Build history of the part. All positions in model axes, mm. Round coordinates to 2 decimals unless told otherwise and drop trailing zeros. Write each loop counter-clockwise with the first axis right and the second up, starting at its lowest first coordinate (ties: lowest second). Pieces come first, ordered by that corner, then holes. Notation, with made-up numbers: (-21.75, -9) -> (20.25, -9) arc R24 ccw to (20.25, 11) -> close; hole circle Ø11 at (67.5, -34.5). An arc over 180 degrees is marked (long way). One line per question, with ' | ' between items.
from build123d import *

# Parameters (mm, degrees)
SKETCH2_R           = 2.4892
SKETCH2_R_2         = 2.489199995
SKETCH2_R_3         = 2.489199998
BOSS_EXTRUDE1_DEPTH = 2.286
FILLET6_R           = 12.7
FILLET7_R           = 15.24


with BuildPart() as part:
    # Sketch2 → Boss-Extrude1 (new body)
    with BuildSketch(Plane.XY):
        Polygon((33.430156219, 560.153270419), (33.430156219, 610.953270419), (-17.369843781, 610.953270419), (-70.882869838, 630.430419049), (-92.601148921, 570.759937623), (-96.944804753, 558.825841343), (-49.208419617, 541.451218062), (-17.464279743, 534.753270419), (33.335720257, 534.753270419), (33.335720257, 547.453270419), align=None)
        with Locations((-4.764279743, 566.503270419)):
            Circle(SKETCH2_R, mode=Mode.SUBTRACT)
        with Locations((-4.764279743, 579.203270419)):
            Circle(SKETCH2_R, mode=Mode.SUBTRACT)
        with Locations((7.935720257, 566.503270419)):
            Circle(SKETCH2_R, mode=Mode.SUBTRACT)
        with Locations((20.635720257, 566.503270419)):
            Circle(SKETCH2_R, mode=Mode.SUBTRACT)
        with Locations((7.935720257, 579.203270419)):
            Circle(SKETCH2_R, mode=Mode.SUBTRACT)
        with Locations((20.635720257, 579.203270419)):
            Circle(SKETCH2_R, mode=Mode.SUBTRACT)
        with Locations((-4.764279743, 591.903270419)):
            Circle(SKETCH2_R, mode=Mode.SUBTRACT)
        with Locations((-4.764279743, 604.603270419)):
            Circle(SKETCH2_R, mode=Mode.SUBTRACT)
        with Locations((7.935720257, 591.903270419)):
            Circle(SKETCH2_R, mode=Mode.SUBTRACT)
        with Locations((20.635720257, 591.903270419)):
            Circle(SKETCH2_R, mode=Mode.SUBTRACT)
        with Locations((7.935720257, 604.603270419)):
            Circle(SKETCH2_R, mode=Mode.SUBTRACT)
        with Locations((20.635720257, 604.603270419)):
            Circle(SKETCH2_R, mode=Mode.SUBTRACT)
        with Locations((20.635720257, 553.803270419)):
            Circle(SKETCH2_R, mode=Mode.SUBTRACT)
        with Locations((-4.764279743, 553.803270419)):
            Circle(SKETCH2_R, mode=Mode.SUBTRACT)
        with Locations((7.935720257, 553.803270419)):
            Circle(SKETCH2_R, mode=Mode.SUBTRACT)
        with Locations((20.635720257, 541.103270419)):
            Circle(SKETCH2_R, mode=Mode.SUBTRACT)
        with Locations((7.935720257, 541.103270419)):
            Circle(SKETCH2_R, mode=Mode.SUBTRACT)
        with Locations((-4.764279743, 541.103270419)):
            Circle(SKETCH2_R, mode=Mode.SUBTRACT)
        with Locations((-37.25240889, 611.432403444)):
            Circle(SKETCH2_R, mode=Mode.SUBTRACT)
        with Locations((-50.283376351, 575.630114592)):
            Circle(SKETCH2_R, mode=Mode.SUBTRACT)
        with Locations((-62.217472635, 579.973770413)):
            Circle(SKETCH2_R, mode=Mode.SUBTRACT)
        with Locations((-74.151568919, 584.317426233)):
            Circle(SKETCH2_R, mode=Mode.SUBTRACT)
        with Locations((-69.80791745, 596.251510539)):
            Circle(SKETCH2_R_2, mode=Mode.SUBTRACT)
        with Locations((-45.93972488, 587.564198905)):
            Circle(SKETCH2_R_2, mode=Mode.SUBTRACT)
        with Locations((-57.873821165, 591.907854722)):
            Circle(SKETCH2_R_2, mode=Mode.SUBTRACT)
        with Locations((-53.530163169, 603.841956995)):
            Circle(SKETCH2_R_3, mode=Mode.SUBTRACT)
        with Locations((-41.596066884, 599.498301178)):
            Circle(SKETCH2_R_3, mode=Mode.SUBTRACT)
        with Locations((-65.464259454, 608.185612812)):
            Circle(SKETCH2_R_3, mode=Mode.SUBTRACT)
        with Locations((-61.120601458, 620.119715085)):
            Circle(SKETCH2_R, mode=Mode.SUBTRACT)
        with Locations((-49.186505174, 615.776059265)):
            Circle(SKETCH2_R, mode=Mode.SUBTRACT)
        with Locations((-78.495224739, 572.383329949)):
            Circle(SKETCH2_R, mode=Mode.SUBTRACT)
        with Locations((-54.627032171, 563.696018308)):
            Circle(SKETCH2_R, mode=Mode.SUBTRACT)
        with Locations((-66.561128455, 568.039674129)):
            Circle(SKETCH2_R, mode=Mode.SUBTRACT)
        with Locations((-58.970687991, 551.761922025)):
            Circle(SKETCH2_R, mode=Mode.SUBTRACT)
        with Locations((-82.838880559, 560.449233665)):
            Circle(SKETCH2_R, mode=Mode.SUBTRACT)
        with Locations((-70.904784275, 556.105577845)):
            Circle(SKETCH2_R, mode=Mode.SUBTRACT)
    extrude(amount=BOSS_EXTRUDE1_DEPTH)

    # Fillet6
    fillet6_edges = [part.edges().sort_by_distance(p)[0] for p in [
        (-70.882869838, 630.430419049, 1.143),
        (-96.944804753, 558.825841343, 1.143),
        (33.430156219, 610.953270419, 1.143),
        (33.335720257, 534.753270419, 1.143),
    ]]
    fillet(fillet6_edges, radius=FILLET6_R - 0.0001)  # a hair under: the kernel refuses the full size

    # Fillet7
    fillet7_edges = [part.edges().sort_by_distance(p)[0] for p in [
        (-17.464279743, 534.753270419, 1.143),
        (-49.208419617, 541.451218062, 1.143),
        (-17.369843781, 610.953270419, 1.143),
    ]]
    fillet(fillet7_edges, radius=FILLET7_R)


solid = part.part
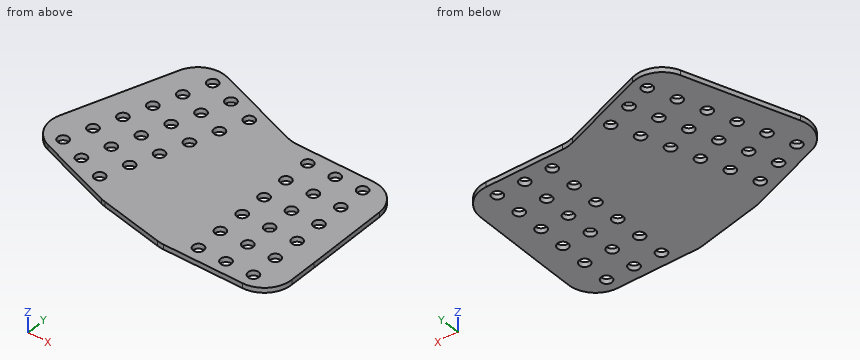
(1) Slice it at C-C (x = -82.5). Write the cut outline in (y, z), then the cut area to 3 significant figures.
Calculated:
outline: (553.57, 0) -> (557.98, 0) -> (557.98, 2.29) -> (553.57, 2.29) -> close; (562.92, 0) -> (598.51, 0) -> (598.51, 2.29) -> (562.92, 2.29) -> close | area: 91.5 mm2
(2) Wall check: line 1 (X direction, y = 603, z = 1.2); line 2 (Y direction, x = -55, z = 0.4); line 3 (Y direction, x = -48, z = 0.85). Give the ranges that are in metal, low to high. Write a range as from..to.
Calculated:
line 1: -80.87..-55.87, -51.19..-6.67, -2.86..6.03, 9.84..18.73, 22.54..32.51 | line 2: 543.56..561.23, 566.16..601.83, 605.85..624.65 | line 3: 541.2..574.64, 576.62..586.17, 588.96..613.59, 617.96..622.1
(3) Slice it at B-B (z = 1.5). State how many separate pieces and enclosed holes the cut face has, then the cut area to 3 significant figures.
Calculated:
separate pieces: 1 | enclosed holes: 36 | area: 8,350 mm2
(4) Slice it at D-D (x = 25). Write the cut outline in (y, z), then the cut area to 3 significant figures.
Calculated:
outline: (535.53, 0) -> (610.21, 0) -> (610.21, 2.29) -> (535.53, 2.29) -> close | area: 171 mm2
(5) Slice it at A-A (x = -41). Write the cut outline in (y, z).
Calculated:
outline: (539.72, 0) -> (597.08, 0) -> (597.08, 2.29) -> (539.72, 2.29) -> close; (601.92, 0) -> (619.55, 0) -> (619.55, 2.29) -> (601.92, 2.29) -> close
(6) Drop a flat-ended pin along its axis: pin 1 (5.5 mm diameter, centred on x = -49.19, y = 615.78, fed in from +Z). Give the stop position or say it passes through.
Calculated:
pin 1: z = 2.29
